Can you work these out from the model? Positions are in its coordinate system, mm. Coordinates: 2 decimals unless noted, no trailing zeros. Write each loop counter-clockwise with the first axis right and the second up, starting at its lowest first coordinate (ties: lowest second). Pieces come first, ordered by that corner, then holes.
```python
from build123d import *

# Parameters (mm, degrees)
SKETCH1_R           = 60
BOSS_EXTRUDE1_DEPTH = 3
SKETCH1_3_R         = 8
BOSS_EXTRUDE2_DEPTH = 5
CUT_EXTRUDE1_REACH  = 10
SKETCH2_R           = 1.5
CUT_EXTRUDE2_REACH  = 5
SKETCH3_R           = 3.75
SKETCH4_R           = 1.5
CUT_EXTRUDE3_DEPTH  = 5


with BuildPart() as part:
    # Sketch1 → Boss-Extrude1 (new body)
    with BuildSketch(Plane(origin=(0, 0, 0), x_dir=(1, 0, 0), z_dir=(0, 1, 0))):
        Circle(SKETCH1_R)
        with BuildLine():
            ThreePointArc((7.5, -53.47663041), (3.660460389, -52.338407931), (2.000000204, -48.694167705))
            Line((2.000000204, -48.694167705), (2.000000204, -16.899494443))
            ThreePointArc((2.000000204, -16.899494443), (6.363961031, -6.363961031), (16.899494443, -2.000000204))
            Line((16.899494443, -2.000000204), (48.694167705, -2.000000204))
            ThreePointArc((48.694167705, -2.000000204), (52.338407931, -3.660460389), (53.47663041, -7.5))
            ThreePointArc((53.47663041, -7.5), (38.183766184, -38.183766184), (7.5, -53.47663041))
        make_face(mode=Mode.SUBTRACT)
        with BuildLine():
            ThreePointArc((53.47663041, 7.5), (52.338407931, 3.660460389), (48.694167705, 2.000000204))
            Line((48.694167705, 2.000000204), (16.899494443, 2.000000204))
            ThreePointArc((16.899494443, 2.000000204), (6.363961031, 6.363961031), (2.000000204, 16.899494443))
            Line((2.000000204, 16.899494443), (2.000000204, 48.694167705))
            ThreePointArc((2.000000204, 48.694167705), (3.660460389, 52.338407931), (7.5, 53.47663041))
            ThreePointArc((7.5, 53.47663041), (38.183766184, 38.183766184), (53.47663041, 7.5))
        make_face(mode=Mode.SUBTRACT)
        with BuildLine():
            ThreePointArc((-7.5, 53.47663041), (-3.660460389, 52.338407931), (-2.000000204, 48.694167705))
            Line((-2.000000204, 48.694167705), (-2.000000204, 16.899494443))
            ThreePointArc((-2.000000204, 16.899494443), (-6.363961031, 6.363961031), (-16.899494443, 2.000000204))
            Line((-16.899494443, 2.000000204), (-48.694167705, 2.000000204))
            ThreePointArc((-48.694167705, 2.000000204), (-52.338407931, 3.660460389), (-53.47663041, 7.5))
            ThreePointArc((-53.47663041, 7.5), (-38.183766184, 38.183766184), (-7.5, 53.47663041))
        make_face(mode=Mode.SUBTRACT)
        with BuildLine():
            ThreePointArc((-53.47663041, -7.5), (-52.338407931, -3.660460389), (-48.694167705, -2.000000204))
            Line((-48.694167705, -2.000000204), (-16.899494443, -2.000000204))
            ThreePointArc((-16.899494443, -2.000000204), (-6.363961031, -6.363961031), (-2.000000204, -16.899494443))
            Line((-2.000000204, -16.899494443), (-2.000000204, -48.694167705))
            ThreePointArc((-2.000000204, -48.694167705), (-3.660460389, -52.338407931), (-7.5, -53.47663041))
            ThreePointArc((-7.5, -53.47663041), (-38.183766184, -38.183766184), (-53.47663041, -7.5))
        make_face(mode=Mode.SUBTRACT)
    extrude(amount=-BOSS_EXTRUDE1_DEPTH)

    # Sketch1<3> → Boss-Extrude2 (add)
    with BuildSketch(Plane(origin=(0, 0, 0), x_dir=(1, 0, 0), z_dir=(0, 1, 0))):
        Circle(SKETCH1_3_R)
    extrude(amount=BOSS_EXTRUDE2_DEPTH)

    # Sketch2 → Cut-Extrude1 (cut, up to next)
    with BuildSketch(Plane(origin=(0, 5, 0), x_dir=(1, 0, 0), z_dir=(0, 1, 0)), mode=Mode.PRIVATE) as cut_extrude1_sk1:
        Circle(SKETCH2_R)
    cut_extrude1_tool1 = extrude(cut_extrude1_sk1.sketch, amount=-CUT_EXTRUDE1_REACH, mode=Mode.PRIVATE) & part.part
    add(cut_extrude1_tool1.solids().sort_by_distance((0, 5, 0))[0], mode=Mode.SUBTRACT)

    # Sketch3 → Cut-Extrude2 (cut, up to next)
    with BuildSketch(Plane(origin=(0, 0, 0), x_dir=(1, 0, 0), z_dir=(0, 1, 0)), mode=Mode.PRIVATE) as cut_extrude2_sk1:
        with Locations((0, -55.25)):
            Circle(SKETCH3_R)
    cut_extrude2_tool1 = extrude(cut_extrude2_sk1.sketch, amount=-CUT_EXTRUDE2_REACH, mode=Mode.PRIVATE) & part.part
    add(cut_extrude2_tool1.solids().sort_by_distance((0, 0, 55.25))[0], mode=Mode.SUBTRACT)

    # Sketch4 → Cut-Extrude3 (cut)
    with BuildSketch(Plane(origin=(0, 5, 0), x_dir=(1, 0, 0), z_dir=(0, 1, 0))):
        with Locations((0, -5.5)):
            Circle(SKETCH4_R)
    extrude(amount=-CUT_EXTRUDE3_DEPTH, mode=Mode.SUBTRACT)


solid = part.part
```
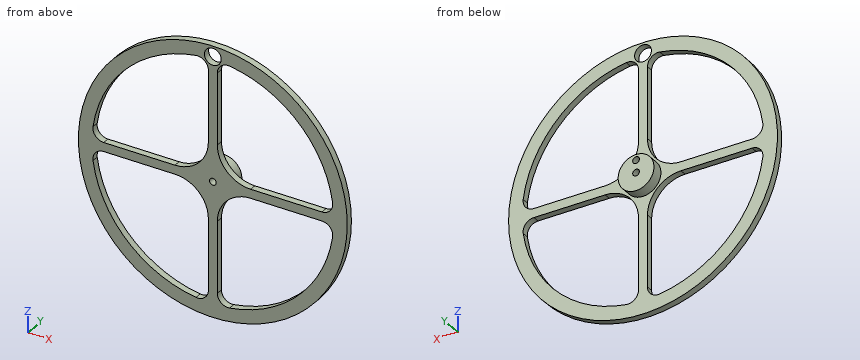
1. If we section it at C-C, the plane z = -41.5: List the corners of the cut face in (x, y) for me.
2. If we section it at B-B, the plane x = 0: List the corners of the cut face in (y, z) for me, plus the area to 4 significant figures.
3. I'm going to push flat-ended pins straight in: P1, Ø2.5, axis at x = 39.5, y = -1.5, coming from the +Z side; P2, Ø1.5, axis at y = -1, z = 35, coming from the -X side; P3, Ø0.9, axis at y = -2, z = -34.5, coming from the +X side. Where does each tip first touch, or does it pass through?
4. If I drill on L1, parallel to Z at x = 0, y = -0.6; L2, parallel to Z at x = 0, y = 3.5; L3, parallel to X at y = -0.25, z = 42, over which ranges is the centre line in solid material (lowest first)?
5. If we section it at A-A, the plane z = 0: List the corners of the cut face in (x, y) for me, plus the area to 3 significant figures.
6. If we section it at D-D, the plane y = 3.5: List the corners of the cut face in (x, z) for me.
Answers:
1. outline: (-43.33, -3) - (-34.55, -3) - (-34.55, 0) - (-43.33, 0) - close; (-2, -3) - (2, -3) - (2, 0) - (-2, 0) - close; (34.55, -3) - (43.33, -3) - (43.33, 0) - (34.55, 0) - close
2. outline: (-3, -60) - (0, -60) - (0, -8) - (5, -8) - (5, -1.5) - (-3, -1.5) - close; (-3, 1.5) - (5, 1.5) - (5, 4) - (0, 4) - (0, 7) - (5, 7) - (5, 8) - (0, 8) - (0, 51.5) - (-3, 51.5) - close; (-3, 59) - (0, 59) - (0, 60) - (-3, 60) - close
2. area: 378.5 mm2
3. P1: stops at z = 46.23
3. P2: stops at x = -49.26
3. P3: stops at x = 49.4
4. L1: z = -60 to -1.5, 1.5 to 51.5, 59 to 60
4. L2: z = -8 to -1.5, 1.5 to 4, 7 to 8
4. L3: x = -42.85 to -33.94, -2 to 2, 33.94 to 42.85
5. outline: (-60, -3) - (-1.5, -3) - (-1.5, 5) - (-8, 5) - (-8, 0) - (-60, 0) - close; (1.5, -3) - (60, -3) - (60, 0) - (8, 0) - (8, 5) - (1.5, 5) - close
5. area: 416 mm2
6. outline: circle Ø16 at (0, 0); hole circle Ø3 at (0, 0); hole circle Ø3 at (0, 5.5)
